Source: CAD feature listing. Evaluate the final solid. Frame: model axes, mm. Face numbers are marked on the shaded views. A direction names the side the tool comes from. Give positions to 0.01 mm unless a question says otherwise; leave off trailing zeros. Order: outer loops, then holes, each group sorted by start corner. A loop starts at its lowest first (then second) coordinate and runs counter-clockwise, first axis right, second up.
```python
from build123d import *

# Parameters (mm, degrees)
SKETCH2_R            = 5
BOSS_EXTRUDE1_DEPTH  = 15
BOSS_EXTRUDE2_DEPTH  = 30
CUT_EXTRUDE1_DEPTH   = 34.911650063
M4_CLEARANCE_HOLE1_D = 4.5
FILLET1_R            = 1
SKETCH8_W            = 18
SKETCH8_H            = 6
SKETCH8_H_2          = 0.659341382
CUT_EXTRUDE2_DEPTH   = 35.727510864
CHAMFER1_SIZE        = 1
FILLET2_R            = 2


with BuildPart() as part:
    # Sketch2 → Boss-Extrude1 (new body)
    with BuildSketch(Plane(origin=(0, 0, 0), x_dir=(1, 0, 0), z_dir=(0, 1, 0))):
        with Locations(Location((0, 0, 0), (0, 0, 270))):
            Circle(SKETCH2_R)
    extrude(amount=BOSS_EXTRUDE1_DEPTH)

    # Sketch3 → Boss-Extrude2 (add)
    with BuildSketch(Plane(origin=(0, 0, 0), x_dir=(0, 0, -1), z_dir=(1, 0, 0))):
        with BuildLine():
            Line((-4, 5), (-4, 10))
            ThreePointArc((-4, 10), (0, 14), (4, 10))
            Line((4, 10), (4, 5))
            ThreePointArc((4, 5), (0, 1), (-4, 5))
        make_face()
    extrude(amount=BOSS_EXTRUDE2_DEPTH)

    # Sketch5 → Cut-Extrude1 (cut, through all)
    with BuildSketch(Plane(origin=(0, 0, 0), x_dir=(1, 0, 0), z_dir=(0, 1, 0))):
        with BuildLine():
            Line((18, 2.2), (25, 2.2))
            ThreePointArc((25, 2.2), (27.2, 0), (25, -2.2))
            Line((25, -2.2), (18, -2.2))
            ThreePointArc((18, -2.2), (15.8, 0), (18, 2.2))
        make_face()
    extrude(amount=CUT_EXTRUDE1_DEPTH, mode=Mode.SUBTRACT)

    # M4 Clearance Hole1 (through all)
    with Locations(Plane(origin=(0, 15, 0), x_dir=(1, 0, 0), z_dir=(0, 1, 0))):
        with Locations((0, 0)):
            Hole(M4_CLEARANCE_HOLE1_D / 2)

    # Fillet1
    fillet1_edges = [part.edges().sort_by_distance(p)[0] for p in [
        (3, 7.5, 4),
        (16.5, 5, 4),
        (3, 7.5, -4),
        (5, 1, 0),
    ]]
    fillet(fillet1_edges, radius=FILLET1_R)

    # Sketch8 → Cut-Extrude2 (cut, through all)
    with BuildSketch(Plane.XY.offset(4)):
        with Locations((21, 7.5)):
            Rectangle(SKETCH8_W, SKETCH8_H)
        with Locations((21, 1.329670691)):
            Rectangle(SKETCH8_W, SKETCH8_H_2)
        with Locations((21, 13.670329309)):
            Rectangle(SKETCH8_W, SKETCH8_H_2)
    extrude(amount=-CUT_EXTRUDE2_DEPTH, mode=Mode.SUBTRACT)

    # Chamfer1
    chamfer1_edges = [part.edges().sort_by_distance(p)[0] for p in [
        (30, 10.5, 0),
        (30, 4.5, 0),
    ]]
    chamfer(chamfer1_edges, length=CHAMFER1_SIZE)

    # Fillet2
    fillet2_edges = [part.edges().sort_by_distance(p)[0] for p in [
        (12, 10.5, 0),
        (12, 4.5, 0),
    ]]
    fillet(fillet2_edges, radius=FILLET2_R)


solid = part.part
```
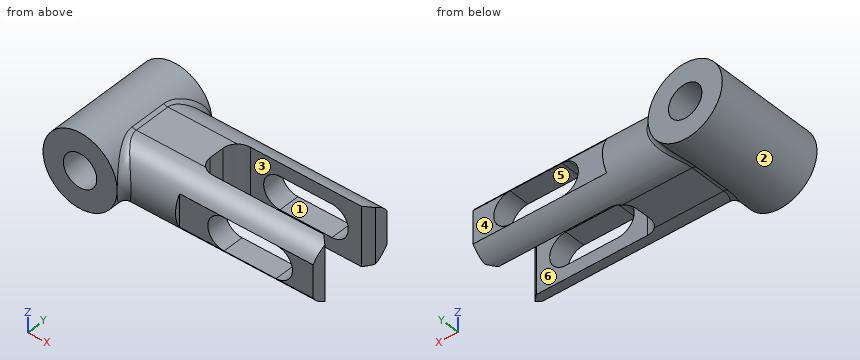
1) Section query A-A, the plane x = 0. Return the cut outline in (y, z).
Report:
outline: (0, -5) - (15, -5) - (15, -2.25) - (0, -2.25) - close; (0, 2.25) - (15, 2.25) - (15, 5) - (0, 5) - close
2) Reachability of the marked faces 4, 5 and 6 from +Z, -Z, +X, -X, +Y, -Y: full face, straight path, thin tool, end or side. Return the list, or none.
Report:
face 4: +Z, -Z, +X, +Y
face 5: +Y, -Y
face 6: +Z, -Z, +X
3) Pin query (flat end, axial travel): pin 1 (4 mm diameter, centred on x = 13, z = -4, fed in from +Y); pin 2 (0.7 mm diameter, centred on y = 14, z = 0.5, fed in from +X); pin 3 (8 mm diameter, centred on x = 12, y = 9.5, fed in from -Z). Return the tip coordinate at first contact, or that it passes through.
Report:
pin 1: stops at y = 13.34
pin 2: stops at x = 12
pin 3: stops at z = -4
4) Section query D-D, the plane z = 0.5. Count the separate pieces of the cut face and the enclosed holes in it, and give its area (3 significant figures).
Report:
separate pieces: 4
enclosed holes: 0
area: 214 mm2
5) Draft query along Z for the marked faces 1, 2 and 3. Return one class per face: +Z half, -Z half, draft (parallel to the pull), parting line (faces both ways), or undercut.
Report:
face 1: undercut
face 2: parting line
face 3: draft
6) Section query B-B, the plane y = 7.5. Return the cut outline in (x, z).
Report:
outline: (2.76, -4.17) arc R1 cw to (3.32, -4) - (12, -4) - (12, 4) - (3.32, 4) arc R1 cw to (2.76, 4.17) arc R5 ccw (long way) to start; hole circle Ø4.5 at (0, 0)
7) Material intervals for L1, parallel to Z at x = 18, y = 11.5; L2, parallel to Y at x = 17, z = 2; L3, parallel to X at y = 3, z = -0.25, sorted ascending.
Report:
L1: z = -3.71 to -2.2, 2.2 to 3.71
L2: y = 1.66 to 4.5, 10.5 to 13.34
L3: x = -4.99 to -2.24, 2.24 to 15.81, 27.19 to 30
8) Section query C-C, the plane x = 17. Return the cut outline in (y, z), and give its area (3 significant figures).
Report:
outline: (1.66, -2.2) arc R4 ccw to (4.5, -3.97) - (4.5, -1.96) - (1.66, -1.96) - close; (1.66, 1.96) - (4.5, 1.96) - (4.5, 3.97) arc R4 ccw to (1.66, 2.2) - close; (10.5, -3.97) arc R4 ccw to (13.34, -2.2) - (13.34, -1.96) - (10.5, -1.96) - close; (10.5, 1.96) - (13.34, 1.96) - (13.34, 2.2) arc R4 ccw to (10.5, 3.97) - close
area: 16.1 mm2
